For this review, take the finished solid that the model builds, in its own axes (mm). Face numbers are marked on the shaded views. A direction names the side the tool comes from. Coordinates: 2 decimals unless noted, no trailing zeros. Write each loop counter-clockwise with the first axis right and the second up, starting at its lowest first coordinate (ties: lowest second). Pieces come first, ordered by that corner, then holes.
```python
from build123d import *

# Parameters (mm, degrees)
F0_W     = 94.439332
F0_H     = 70.08286
F1_DEPTH = 44.45
F2_R     = 20.277827
F3_DEPTH = 25.4
F4_R     = 10.364463
F5_DEPTH = 69.85


with BuildPart() as f1:
    # F0 (on Front) → F1 (new body)
    with BuildSketch(Plane.XZ):
        with Locations((2.542602, -3.987971)):
            Rectangle(F0_W, F0_H)
    extrude(amount=F1_DEPTH)

    # F2 (on face) → F3 (join)
    with BuildSketch(Plane.XZ.offset(44.45)):
        Circle(F2_R)
    extrude(amount=F3_DEPTH)

    # F4 (on face) → F5 (cut, through all)
    with BuildSketch(Plane.XZ.offset(69.85)):
        Circle(F4_R)
    extrude(amount=-F5_DEPTH, mode=Mode.SUBTRACT)


solid = f1.part
```
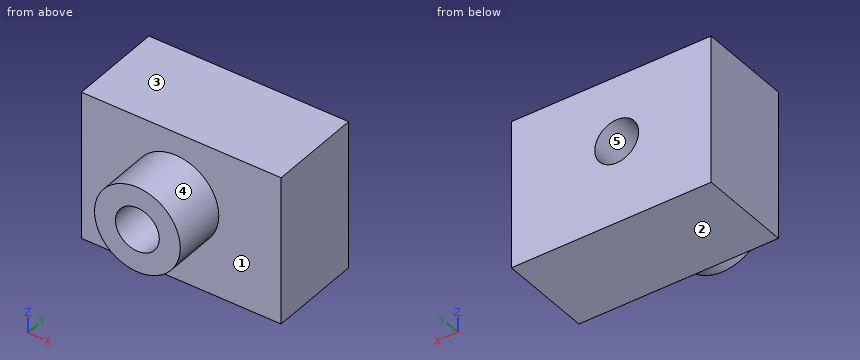
Q1. Draft analysis for pull direction X (two halves, no side actions). For the marked faces 3, 4 and 5, state which applies: +X half, -X half, draft (parallel to the pull), parting line (faces both ways), or undercut.
Ans:
face 3: draft
face 4: parting line
face 5: undercut
Q2. Add section D-D (x = 22). State the section outline as (y, z) points.
Ans:
outline: (-44.45, -39.03) - (0, -39.03) - (0, 31.05) - (-44.45, 31.05) - close
Q3. Clearance check with flat-ended pins moving along their axes: pin 1 Ø3 at (x, y) = (3, -52) entering from +Z; pin 2 Ø4 at (x, z) = (30.5, -17) entering from -Y; pin 3 Ø3 at (x, z) = (15, -15.5) entering from +Y. State where each tip first meets the part, or that it passes through.
Ans:
pin 1: stops at z = 20.22
pin 2: stops at y = -44.45
pin 3: stops at y = 0
Q4. Tool access review of the marked faces 1 and 2: name each direction out of +Z, -Z, +X, -X, +Y, -Y from which nothing blocks a thin tool from reaching the whole face with its end or side.
Ans:
face 1: -Y
face 2: -Z, +X, -X, +Y, -Y
Q5. Add section B-B (z = 0). State the section outline as (x, y) points, then the cut area to 3 significant figures.
Ans:
outline: (-44.68, -44.45) - (-20.28, -44.45) - (-20.28, -69.85) - (-10.36, -69.85) - (-10.36, 0) - (-44.68, 0) - close; (10.36, -69.85) - (20.28, -69.85) - (20.28, -44.45) - (49.76, -44.45) - (49.76, 0) - (10.36, 0) - close
area: 3,780 mm2
Q6. For probe 1 along Z at (x, y) = (0, -30); probe 2 along Z at (x, y) = (0, -45.5); probe 3 along Y at (x, z) = (-24.5, -29), list the stretches that pass through material, from the lowest coordinate up.
Ans:
probe 1: z = -39.03 to -10.36, 10.36 to 31.05
probe 2: z = -20.28 to -10.36, 10.36 to 20.28
probe 3: y = -44.45 to 0
Q7. Add section C-C (y = -27). State the section outline as (x, z) points, then the cut area to 3 significant figures.
Ans:
outline: (-44.68, -39.03) - (49.76, -39.03) - (49.76, 31.05) - (-44.68, 31.05) - close; hole circle Ø20.73 at (0, 0)
area: 6,280 mm2
Q8. Add section A-A (x = 0). State the section outline as (y, z) points.
Ans:
outline: (-69.85, -20.28) - (-44.45, -20.28) - (-44.45, -39.03) - (0, -39.03) - (0, -10.36) - (-69.85, -10.36) - close; (-69.85, 10.36) - (0, 10.36) - (0, 31.05) - (-44.45, 31.05) - (-44.45, 20.28) - (-69.85, 20.28) - close
